from build123d import *

# Parameters (mm, degrees)
SKETCH1_W           = 4
SKETCH1_H           = 4
SKETCH1_R           = 3.7500052
BOSS_EXTRUDE1_DEPTH = 1.2
SKETCH1_5_W         = 16
SKETCH1_5_H         = 5
SKETCH1_5_W_2       = 10
BOSS_EXTRUDE3_DEPTH = 0.6


with BuildPart() as part:
    # Sketch1 → Boss-Extrude1 (new body)
    with BuildSketch(Plane(origin=(0, 0, 0), x_dir=(1, 0, 0), z_dir=(0, 1, 0))):
        Polygon((-25, -30), (-25, -40), (25, -40), (25, -32), (15, -32), (15, -27), (25, -27), (25, 8), (-25, 8), (-25, -25), (-9, -25), (-9, -30), align=None)
        with Locations((0, -30)):
            Rectangle(SKETCH1_W, SKETCH1_H, mode=Mode.SUBTRACT)
        with Locations(Location((-18.5, 0, 0), (0, 0, 270))):
            Circle(SKETCH1_R, mode=Mode.SUBTRACT)
        with Locations(Location((0, 0, 0), (0, 0, 270))):
            Circle(SKETCH1_R, mode=Mode.SUBTRACT)
        with Locations(Location((18.5, 0, 0), (0, 0, 270))):
            Circle(SKETCH1_R, mode=Mode.SUBTRACT)
    extrude(amount=BOSS_EXTRUDE1_DEPTH)

    # Sketch1_5 → Boss-Extrude3 (add)
    with BuildSketch(Plane(origin=(0, 0, 0), x_dir=(1, 0, 0), z_dir=(0, 1, 0))):
        with Locations((-17, -27.5)):
            Rectangle(SKETCH1_5_W, SKETCH1_5_H)
        with Locations((20, -29.5)):
            Rectangle(SKETCH1_5_W_2, SKETCH1_5_H)
    extrude(amount=BOSS_EXTRUDE3_DEPTH)


solid = part.part
The listing builds one solid part. Answer for the finished solid, in the listing's coordinates (mm). A direction names the side the tool comes from. Give positions to 0.01 mm unless a question says otherwise; leave off trailing zeros. Write each loop counter-clockwise with the first axis right and the second up, starting at its lowest first coordinate (ties: lowest second). Pieces come first, ordered by that corner, then holes.
1) Section C-C (x = 0) is taken. Write down the section's boundary in (y, z), and give its area (3 significant figures).
2) Section B-B (y = 0.3) is taken. Write down the section's boundary in (x, z).
3) For a pull along Z with two mould halves and no side action, classify faces 1 (the face through (0, 1, 40)), 2 (the face through (-14.782, 0.592, -0.488)), 3 (the face through (0, 1.2, 16)) as pulls with the +Z half, pulls with the -Z half, needs draft (parallel to the pull), parting line crosses it, or undercut.
4) Section D-D (x = -14) is taken. Write down the section's boundary in (y, z), and give its area (3 significant figures).
5) Find the intervals of material crossed by L1, parallel to X at y = 0.3, z = 0; L2, parallel to X at y = 0.85, z = 29; L3, parallel to X at y = 0.35, z = 29.5, in increasing order.
6) Section A-A (z = 0) is taken. Write down the section's boundary in (x, y), and give its area (3 significant figures).
7) Given P1, Ø4, axis at x = -18, z = -2.5, coming from the -Y side; P2, Ø1.5, axis at x = -20.5, z = 27.5, coming from the +Y side, each flat-ended and moving along its own axis, determine where each tip first touches the part or whether it passes through.
8) A tool of negligible diameter and unlimited length cuts with its end or side. For faces 4 (the face through (20, 0.6, 29)), 5 (the face through (0, 1, 28)), 6 (the face through (-17, 0.6, 27)), from which of +Z, -Z, +X, -X, +Y, -Y can it reach the whole face along a straight path? Write none if from no direction.
Response:
1. outline: (0, -8) - (1.2, -8) - (1.2, -3.75) - (0, -3.75) - close; (0, 3.75) - (1.2, 3.75) - (1.2, 28) - (0, 28) - close; (0, 32) - (1.2, 32) - (1.2, 40) - (0, 40) - close
1. area: 43.8 mm2
2. outline: (-25, -8) - (25, -8) - (25, 40) - (-25, 40) - close; hole circle Ø7.5 at (-18.5, 0); hole circle Ø7.5 at (0, 0); hole (-2, 28) - (2, 28) - (2, 32) - (-2, 32) - close; hole circle Ø7.5 at (18.5, 0)
3. face 1: pulls with the +Z half
3. face 2: undercut
3. face 3: needs draft
4. outline: (0, -8) - (1.2, -8) - (1.2, 25) - (0.6, 25) - (0.6, 30) - (1.2, 30) - (1.2, 40) - (0, 40) - close
4. area: 54.6 mm2
5. L1: x = -25 to -22.25, -14.75 to -3.75, 3.75 to 14.75, 22.25 to 25
5. L2: x = -9 to -2, 2 to 15
5. L3: x = -25 to -2, 2 to 25
6. outline: (-25, 0) - (-22.25, 0) - (-22.25, 1.2) - (-25, 1.2) - close; (-14.75, 0) - (-3.75, 0) - (-3.75, 1.2) - (-14.75, 1.2) - close; (3.75, 0) - (14.75, 0) - (14.75, 1.2) - (3.75, 1.2) - close; (22.25, 0) - (25, 0) - (25, 1.2) - (22.25, 1.2) - close
6. area: 33.0 mm2
7. P1: stops at y = 0
7. P2: stops at y = 0.6
8. face 4: +X, +Y
8. face 5: +Y, -Y
8. face 6: -X, +Y
